Design review of the part built by this model. Coordinates are the model's own, in mm. A direction names the side the tool comes from. Coordinates: 2 decimals unless noted, no trailing zeros. Loops run counter-clockwise (first coordinate to the right, second up) from the corner with the lowest first, then second, coordinate; pieces in that order, holes last. Notation, with made-up numbers: M 69.25,24.5 L 121.25,24.5 A22 ccw 121.25,59.5 Z; hole C 9.25,13 d1. An arc over 180 degrees is marked long. Write item = value, one per line. Start each with the question number.
from build123d import *

# Parameters (mm, degrees)
SKETCH1_W                                    = 51.7
SKETCH1_H                                    = 1.875
SKETCH2_W                                    = 3
SKETCH2_H                                    = 3.625
CHAMFER1_SIZE                                = 1
M2_CLEARANCE_HOLE1_D                         = 2.4
M2_CLEARANCE_HOLE1_DEPTH                     = 11.5
CIRPATTERN1_COUNT                            = 6
SKETCH6_W                                    = 3
SKETCH6_H                                    = 19
REVOLVE3_ANGLE                               = 135
SKETCH9_W                                    = 3
SKETCH9_H                                    = 8
CHAMFER2_SIZE                                = 0.5
SKETCH11_W                                   = 5
SKETCH11_H                                   = 6
REVOLVE5_ANGLE                               = 135
CHAMFER4_SIZE                                = 1
TAP_DRILL_FOR_M1_6_TAP1_D                    = 1.25
TAP_DRILL_FOR_M1_6_TAP1_DEPTH                = 11.5
CIRPATTERN2_COUNT                            = 12
FILLET1_R                                    = 2
SKETCH17_W                                   = 2.5
SKETCH17_H                                   = 1.95
ESQUISSE2_W                                  = 1
ESQUISSE2_H                                  = 6
R_VOLUTION4_ANGLE                            = 135
SKETCH13_W                                   = 0.8
SKETCH13_H                                   = 41.8
TROU_POUR_TARAUDAGE_POUR_TROU_TARAUD_2_COUNT = 2
TROU_POUR_TARAUDAGE_POUR_TROU_TARAUD_2_PITCH = 11.563340196
TROU_POUR_TARAUDAGE_POUR_TROU_TARAUD_3_COUNT = 2
TROU_POUR_TARAUDAGE_POUR_TROU_TARAUD_3_PITCH = 11.563340196
TROU_POUR_TARAUDAGE_POUR_TROU_TARAUD_4_COUNT = 2
TROU_POUR_TARAUDAGE_POUR_TROU_TARAUD_4_PITCH = 22.662405452
TROU_POUR_TARAUDAGE_POUR_TROU_TARAUD_5_COUNT = 2
TROU_POUR_TARAUDAGE_POUR_TROU_TARAUD_5_PITCH = 32.851561742
TROU_POUR_TARAUDAGE_POUR_TROU_TARAUD_6_COUNT = 2
TROU_POUR_TARAUDAGE_POUR_TROU_TARAUD_6_PITCH = 41.72170842


with BuildPart() as part:
    # Sketch1 → Revolve1 (revolve)
    with BuildSketch(Plane.XY):
        with Locations((-14.45, 12.0625)):
            Rectangle(SKETCH1_W, SKETCH1_H)
    revolve(axis=Axis((0, 0, 0), (1, 0, 0)))

    # Sketch2 → Revolve2 (revolve)
    with BuildSketch(Plane.XY):
        with Locations((-38.8, 9.3125)):
            Rectangle(SKETCH2_W, SKETCH2_H)
    revolve(axis=Axis((-40.3, 0, 0), (1, 0, 0)))

    # Chamfer1
    chamfer1_edges = [part.edges().sort_by_distance(p)[0] for p in [
        (-40.3, -13, 0),
    ]]
    chamfer(chamfer1_edges, length=CHAMFER1_SIZE)

    # M2 Clearance Hole1
    with Locations(Plane.ZY.offset(40.3)):
        with Locations((0, 9.5)):
            m2_clearance_hole1 = Hole(M2_CLEARANCE_HOLE1_D / 2, depth=M2_CLEARANCE_HOLE1_DEPTH)

    # CirPattern1: M2 Clearance Hole1 ×6 about axis
    cirpattern1_axis = Axis((0, 0, 0), (1, 0, 0))
    for i in range(1, CIRPATTERN1_COUNT):
        add(m2_clearance_hole1.rotate(cirpattern1_axis, i * 360 / CIRPATTERN1_COUNT), mode=Mode.SUBTRACT)

    # Sketch6 → Revolve3 (revolve, symmetric)
    with BuildSketch(Plane.XY) as revolve3_sk:
        with Locations((0, 22.5)):
            Rectangle(SKETCH6_W, SKETCH6_H)
    revolve(axis=Axis((0, 0, 0), (1, 0, 0)), revolution_arc=REVOLVE3_ANGLE / 2)
    revolve(revolve3_sk.sketch, axis=Axis((0, 0, 0), (-1, 0, 0)), revolution_arc=REVOLVE3_ANGLE / 2)

    # Sketch9 → Revolve4 (revolve)
    with BuildSketch(Plane.XY):
        with Locations((0, 17)):
            Rectangle(SKETCH9_W, SKETCH9_H)
    revolve(axis=Axis((0, 0, 0), (1, 0, 0)))

    # Chamfer2
    chamfer2_edges = [part.edges().sort_by_distance(p)[0] for p in [
        (-1.5, -13, 0),
        (1.5, -13, 0),
    ]]
    chamfer(chamfer2_edges, length=CHAMFER2_SIZE)

    # Sketch11 → Revolve5 (revolve, symmetric)
    with BuildSketch(Plane.XY) as revolve5_sk:
        with Locations((-1, 29)):
            Rectangle(SKETCH11_W, SKETCH11_H)
    revolve(axis=Axis((0, 0, 0), (1, 0, 0)), revolution_arc=REVOLVE5_ANGLE / 2)
    revolve(revolve5_sk.sketch, axis=Axis((0, 0, 0), (-1, 0, 0)), revolution_arc=REVOLVE5_ANGLE / 2)

    # Chamfer4
    chamfer4_edges = [part.edges().sort_by_distance(p)[0] for p in [
        (-3.5, 32, 0),
    ]]
    chamfer(chamfer4_edges, length=CHAMFER4_SIZE)

    # Tap Drill for M1.6 Tap1
    with Locations(Plane.ZY.offset(1.5)):
        with Locations((0, 17.5)):
            tap_drill_for_m1_6_tap1 = Hole(TAP_DRILL_FOR_M1_6_TAP1_D / 2, depth=TAP_DRILL_FOR_M1_6_TAP1_DEPTH)

    # CirPattern2: Tap Drill for M1.6 Tap1 ×12 about axis
    cirpattern2_axis = Axis((0, 0, 0), (1, 0, 0))
    for i in range(1, CIRPATTERN2_COUNT):
        add(tap_drill_for_m1_6_tap1.rotate(cirpattern2_axis, i * 360 / CIRPATTERN2_COUNT), mode=Mode.SUBTRACT)

    # Fillet1
    fillet1_edges = [part.edges().sort_by_distance(p)[0] for p in [
        (0, 8.03635208, -19.401470183),
        (0, 8.03635208, 19.401470183),
    ]]
    fillet(fillet1_edges, radius=FILLET1_R)

    # Sketch17 → Revolve6 (revolve)
    with BuildSketch(Plane.XY):
        with Locations((-5.55, 13.975)):
            Rectangle(SKETCH17_W, SKETCH17_H)
    revolve(axis=Axis((0, 0, 0), (-1, 0, 0)))

    # Esquisse1 → Enlèvement de matière-Révolution1 (revolve, cut)
    with BuildSketch(Plane(origin=(0, 0, 0), x_dir=(1, 0, 0), z_dir=(0, -0.923879533, 0.382683432))):
        Polygon((-3.5, 31), (-2.5, 32), (-2.5, 26), (-3.5, 26), align=None)
    revolve(axis=Axis((-40.3, 0, 0), (1, 0, 0)), mode=Mode.SUBTRACT)

    # Esquisse2 → Révolution4 (revolve)
    with BuildSketch(Plane(origin=(0, 0, 0), x_dir=(1, 0, 0), z_dir=(0, -0.923879533, 0.382683432))):
        with Locations((2, 29)):
            Rectangle(ESQUISSE2_W, ESQUISSE2_H)
    revolve(axis=Axis((11.4, 0, 0), (-1, 0, 0)), revolution_arc=R_VOLUTION4_ANGLE)

    # Sketch13 → Trou pour taraudage pour trou taraudé M21 (revolve, cut)
    with BuildSketch(Plane(origin=(1.5, 23.89965947, -16.425780871), x_dir=(0, 0, -1), z_dir=(0, 1, 0))):
        with Locations((0.4, 19.9)):
            Rectangle(SKETCH13_W, SKETCH13_H)
    trou_pour_taraudage_pour_trou_taraud_m2 = revolve(axis=Axis((8.85, 23.89965947, -16.425780871), (-1, 0, 0)), mode=Mode.SUBTRACT)

    # Trou pour taraudage pour trou taraud 2: Trou pour taraudage pour trou taraudé M21 ×2
    with Locations(*[Vector(0, -0.7193398, -0.69465837) * (i * TROU_POUR_TARAUDAGE_POUR_TROU_TARAUD_2_PITCH) for i in range(1, TROU_POUR_TARAUDAGE_POUR_TROU_TARAUD_2_COUNT)]):
        add(trou_pour_taraudage_pour_trou_taraud_m2, mode=Mode.SUBTRACT)

    # Trou pour taraudage pour trou taraud 3: Trou pour taraudage pour trou taraudé M21 ×2
    with Locations(*[Vector(0, 0.390731128, 0.920504853) * (i * TROU_POUR_TARAUDAGE_POUR_TROU_TARAUD_3_PITCH) for i in range(1, TROU_POUR_TARAUDAGE_POUR_TROU_TARAUD_3_COUNT)]):
        add(trou_pour_taraudage_pour_trou_taraud_m2, mode=Mode.SUBTRACT)

    # Trou pour taraudage pour trou taraud 4: Trou pour taraudage pour trou taraudé M21 ×2
    with Locations(*[Vector(0, 0.199367934, 0.979924705) * (i * TROU_POUR_TARAUDAGE_POUR_TROU_TARAUD_4_PITCH) for i in range(1, TROU_POUR_TARAUDAGE_POUR_TROU_TARAUD_4_COUNT)]):
        add(trou_pour_taraudage_pour_trou_taraud_m2, mode=Mode.SUBTRACT)

    # Trou pour taraudage pour trou taraud 5: Trou pour taraudage pour trou taraudé M21 ×2
    with Locations(*[(0, 0, i * TROU_POUR_TARAUDAGE_POUR_TROU_TARAUD_5_PITCH) for i in range(1, TROU_POUR_TARAUDAGE_POUR_TROU_TARAUD_5_COUNT)]):
        add(trou_pour_taraudage_pour_trou_taraud_m2, mode=Mode.SUBTRACT)

    # Trou pour taraudage pour trou taraud 6: Trou pour taraudage pour trou taraudé M21 ×2
    with Locations(*[Vector(0, -0.199367934, 0.979924705) * (i * TROU_POUR_TARAUDAGE_POUR_TROU_TARAUD_6_PITCH) for i in range(1, TROU_POUR_TARAUDAGE_POUR_TROU_TARAUD_6_COUNT)]):
        add(trou_pour_taraudage_pour_trou_taraud_m2, mode=Mode.SUBTRACT)


solid = part.part
Q1. Add section C-C on y = -4.75. Give the number of separate pieces and of enclosed holes in the cut face, plus the area to 3 significant figures.
Q2. Mouldability with a two-part tool opening along X and no side actions: class faces 4 (the face through (-37.3, -7.3, -2.3)), 5 (the face through (6.766, -10.316, -7.91)), 6 (the face through (-1.5, 13, 5)) as released by +X, released by -X, zero draft, split by the parting line, or undercut.
Q3. Add section A-A on x = -29. State the section outline as (y, z) points (3 decimals), plus the area to 3 significant figures.
Q4. To check wall thickness, follow line 1 (Z direction, x = -5, y = 0) (3 decimals); line 2 (Z direction, x = -25, y = 0) (3 decimals); line 3 (Y direction, x = -36.5, z = -7). State the ranges of each line that lie inside material, in increasing order. Write a range as from..to.
Q5. Add section B-B on y = 21.5. State the section outline as (x, z) points, plus the area to 3 significant figures.
Q6. Clearance check with flat-ended pins moving along their axes: P1, Ø17.5, axis at y = 23, z = -10, coming from the +X side; P2, Ø2, axis at x = -2, y = 5, coming from the -Z side; P3, Ø8, axis at x = -5.5, z = -21.5, coming from the +Y side. State where each tip first meets the part, or that it passes through.
Q7. For faces 1 (the face through (-0.035, 27.625, -5.678)), 2 (the face through (-4.3, 0.1, -13.4)), 3 (the face through (-2, 26, 0)), list the 3-axis set-ups (+Z, -Z, +X, -X, +Y, -Y) from which the entire face can be reached by the end or side of a thin tool; tool diameter is ignored.
Values follow:
q1.separate_pieces = 4
q1.enclosed_holes = 0
q1.area = 282 mm2
q2.face_4 = released by +X
q2.face_5 = zero draft
q2.face_6 = undercut
q3.outline = C 0,0 d26; hole C 0,0 d22.25
q3.area = 142 mm2
q4.line_1 = -14.95..-11.125, 11.125..14.95
q4.line_2 = -13..-11.125, 11.125..13
q4.line_3 = -10.95..-8.65, 8.65..10.95
q5.outline = M -2.5,-23.7 L 2.5,-23.7 L 2.5,-14.62 L 1.5,-14.62 L 1.5,14.62 L 2.5,14.62 L 2.5,23.7 L -2.5,23.7 L -2.5,14.62 L -1.5,14.62 L -1.5,-14.62 L -2.5,-14.62 Z
q5.area = 179 mm2
q6.P1 = 2.5
q6.P2 = -20.59
q6.P3 = 25.86
q7.face_1 = +X, -X
q7.face_2 = none
q7.face_3 = -X
